```python
from build123d import *

# Parameters (mm, degrees)
F0_R     = 12.7
F1_DEPTH = 60.325
F2_DEPTH = 19.05
F3_DEPTH = 19.05
F4_R     = 5.08
F5_R     = 6.35
F6_DEPTH = 25.4


with BuildPart() as f1:
    # F0 (on Front) → F1 (new body)
    with BuildSketch(Plane.XZ):
        with BuildLine():
            ThreePointArc((-55.109176, 0), (-39.303925, 6.546749), (-32.757176, 22.352))
            ThreePointArc((-32.757176, 22.352), (-70.914426, 38.157251), (-55.109176, 0))
        make_face()
        with Locations((-55.109176, 22.352)):
            Circle(F0_R, mode=Mode.SUBTRACT)
        with BuildLine():
            Line((30.742824, 22.352), (-32.757176, 22.352))
            ThreePointArc((-32.757176, 22.352), (-39.303925, 6.546749), (-55.109176, 0))
            Line((-55.109176, 0), (36.737224, 0))
            Line((36.737224, 0), (30.742824, 22.352))
        make_face()
        Polygon((62.137224, 22.352), (30.742824, 22.352), (36.737224, 0), (62.137224, 0), align=None)
        with BuildLine():
            Line((94.979424, 22.352), (62.137224, 22.352))
            Line((62.137224, 22.352), (62.137224, 0))
            Line((62.137224, 0), (139.099224, 0))
            Line((139.099224, 0), (139.099224, 14.478))
            ThreePointArc((139.099224, 14.478), (136.792983, 20.045759), (131.225224, 22.352))
            Line((131.225224, 22.352), (94.979424, 22.352))
        make_face()
    extrude(amount=-F1_DEPTH)

    # F0 (on Front) → F2 (join)
    with BuildSketch(Plane.XZ):
        with BuildLine():
            ThreePointArc((75.929424, 57.15), (72.35524, 38.434358), (62.137224, 22.352))
            Line((62.137224, 22.352), (94.979424, 22.352))
            Line((94.979424, 22.352), (94.979424, 52.07))
            ThreePointArc((94.979424, 52.07), (93.491527, 55.662102), (89.899424, 57.15))
            Line((89.899424, 57.15), (75.929424, 57.15))
        make_face()
    extrude(amount=-F2_DEPTH)

    # F0 (on Front) → F3 (cut)
    with BuildSketch(Plane.XZ):
        Polygon((62.137224, 22.352), (30.742824, 22.352), (36.737224, 0), (62.137224, 0), align=None)
    extrude(amount=-F3_DEPTH, mode=Mode.SUBTRACT)

    # F4
    f4_edges = [f1.edges().sort_by_distance(p)[0] for p in [
        (-32.757176, 30.1625, 22.352),
        (94.979424, 9.525, 22.352),
    ]]
    fillet(f4_edges, radius=F4_R)

    # F5 (on face) → F6 (cut)
    with BuildSketch(Plane.XY.offset(22.352)):
        with Locations((100.237224, 37.973)):
            Circle(F5_R)
    extrude(amount=-F6_DEPTH, mode=Mode.SUBTRACT)


solid = f1.part
```
CAD build for the part. Positions are in the model's coordinates, mm. A direction names the side the tool comes from. Give positions to 0.01 mm unless a question says otherwise; leave off trailing zeros. Write each loop counter-clockwise with the first axis right and the second up, starting at its lowest first coordinate (ties: lowest second). Pieces come first, ordered by that corner, then holes. Notation, with made-up numbers: M 29.25,-23 L 39.25,-23 A17 cw 39.25,-16 Z; hole C 7.25,28.25 d2. An arc over 180 degrees is marked long. Return JSON: item names as keys, results as strings. Group by question number.
(1) Flat gauge pins, fed straight in: pin 1 Ø6 at (y, z) = (40.5, 21.5) entering from -X; pin 2 Ø2 at (y, z) = (24, 13) entering from -X; pin 3 Ø4 at (y, z) = (35.5, 22) entering from +X; pin 4 Ø15 at (y, z) = (10.5, 7.5) entering from -X. Where does each tip first touch, or does it go through?
(2) Band-saw the part on C-C (z = 12). Give the cut face in (x, y) (3 decimals).
(3) Drill centre lines: L1, parallel to X at y = 14, z = 18; L2, parallel to X at y = 7.5, z = 19.5; L3, parallel to Z at x = 47.5, y = 28.5. Where is each one in solid material? Low to high. Write a range as [from, to].
(4) Band-saw the part on D-D (x = 112). Give the cut face in (y, z) (3 decimals), and give its area (3 significant figures).
(5) Band-saw the part on A-A (y = 4). Give the cut face in (x, z), and give its area (3 significant figures).
(6) Band-saw the part on B-B (y = 24.5). Give the cut face in (x, z), and give its area (3 significant figures).
(7) 3-axis set-ups, long thin cutter, end or side, ignore diameter. For faces 4 (the face through (62.137, 9, 11)), 5 (the face through (46, 19.05, 11)), 6 (the face through (-31.43, 30.58, 23.55)): which of +Z, -Z, +X, -X, +Y, -Y reach the whole face in a straight line?
(8) Mould opens along Z. For faces 1 (the face through (-64.5, 29.7, 30.9)), 2 (the face through (72.45, 9.39, 38.68)), 3 (the face through (92, 0, 23)) say: pulls with the +Z half, pulls with the -Z half, needs draft (parallel to the pull), parting line crosses it, or undercut.
Entries:
{
 "1": {"pin 1": "stops at x = -77.46", "pin 2": "stops at x = -75.84", "pin 3": "stops at x = 136.84", "pin 4": "stops at x = -76.22"},
 "2": {"outline": "M -74.919,0 L -62.466,0 L -62.466,60.325 L -74.919,60.325 Z; M -47.752,0 L 33.519,0 L 33.519,19.05 L 62.137,19.05 L 62.137,0 L 139.099,0 L 139.099,60.325 L -47.752,60.325 Z; hole C 100.237,37.973 d12.7"},
 "3": {"L1": "x = [-77.03, -67.04], [-43.18, 31.91], [62.14, 138.27]", "L2": "x = [-77.28, -67.48], [-42.73, 31.51], [62.14, 137.29]", "L3": "z = [0, 22.35]"},
 "4": {"outline": "M 0,0 L 60.325,0 L 60.325,22.352 L 0,22.352 Z", "area": "1,350 mm^2"},
 "5": {"outline": "M -55.11,0 L 36.74,0 L 30.74,22.35 L -28.15,22.35 A5.08 cw -33.14,26.49 A22.35 ccw long Z; M 62.14,0 L 139.1,0 L 139.1,14.48 A7.87 ccw 131.23,22.35 L 100.06,22.35 A5.08 cw 94.98,27.43 L 94.98,52.07 A5.08 ccw 89.9,57.15 L 75.93,57.15 A50.8 cw 62.14,22.35 Z; hole C -55.11,22.35 d25.4", "area": "5,180 mm^2"},
 "6": {"outline": "M -55.11,0 L 139.1,0 L 139.1,14.48 A7.87 ccw 131.23,22.35 L -28.15,22.35 A5.08 cw -33.14,26.49 A22.35 ccw long Z; hole C -55.11,22.35 d25.4", "area": "5,000 mm^2"},
 "7": {"face 4": "+Z, -Z, -Y", "face 5": "+Z, -Y", "face 6": "+Z, +Y, -Y"},
 "8": {"face 1": "undercut", "face 2": "pulls with the +Z half", "face 3": "needs draft"}
}
